```python
from build123d import *

# Parameters (mm, degrees)
BOSS_EXTRU_2_DEPTH      = 73
ESQUISSE6_W             = 6
ESQUISSE6_H             = 5
ENL_V_MAT_EXTRU_3_DEPTH = 83.675570757
ESQUISSE7_R             = 1.75
ENL_V_MAT_EXTRU_4_DEPTH = 12
ENL_V_START             = -12
ESQUISSE8_R             = 1.75
ENL_V_MAT_EXTRU_5_DEPTH = 12
CONG_1_R                = 3
ENL_V_START_2           = -3
ENL_V_MAT_EXTRU_6_DEPTH = 2.6
ENL_V_START_3           = -5.6
ENL_V_MAT_EXTRU_7_DEPTH = 2.6


with BuildPart() as part:
    # Esquisse3 → Boss.-Extru.2 (new body)
    with BuildSketch(Plane.XY):
        with BuildLine():
            ThreePointArc((-5, 37.165171868), (0, 37.5), (5, 37.165171868))
            Line((5, 37.165171868), (5, 29.580398915))
            Line((5, 29.580398915), (-5, 29.580398915))
            Line((-5, 29.580398915), (-5, 37.165171868))
        make_face()
    extrude(amount=BOSS_EXTRU_2_DEPTH)

    # Esquisse6 → Enlèv. mat.-Extru.3 (cut, through all)
    with BuildSketch(Plane.ZY.offset(5)):
        with Locations((18, 37.080398915)):
            Rectangle(ESQUISSE6_W, ESQUISSE6_H)
        with Locations((55, 37.080398915)):
            Rectangle(ESQUISSE6_W, ESQUISSE6_H)
    extrude(amount=-ENL_V_MAT_EXTRU_3_DEPTH, mode=Mode.SUBTRACT)

    # Esquisse7 → Enlèv. mat.-Extru.4 (cut)
    with BuildSketch(Plane.XY.offset(73)):
        with Locations((0, 33.75)):
            Circle(ESQUISSE7_R)
    extrude(amount=-ENL_V_MAT_EXTRU_4_DEPTH, mode=Mode.SUBTRACT)

    # Esquisse8 → Enlèv. mat.-Extru.5 (cut)
    with BuildSketch(Plane(origin=(0, 0, 0), x_dir=(-1, 0, 0), z_dir=(0, 0, -1)).offset(ENL_V_START)):
        with Locations(Location((0, 33.75, 0), (0, 0, 180))):
            Circle(ESQUISSE8_R)
    extrude(amount=ENL_V_MAT_EXTRU_5_DEPTH, mode=Mode.SUBTRACT)

    # Congé1
    cong_1_edges = [part.edges().sort_by_distance(p)[0] for p in [
        (5, 34.580398915, 18),
        (-5, 34.580398915, 18),
        (5, 34.580398915, 55),
        (-5, 34.580398915, 55),
    ]]
    fillet(cong_1_edges, radius=CONG_1_R)

    # Esquisse9 → Enlèv. mat.-Extru.6 (cut)
    with BuildSketch(Plane(origin=(0, 0, 0), x_dir=(-1, 0, 0), z_dir=(0, 0, -1)).offset(ENL_V_START_2)):
        with BuildLine():
            Line((-2.85, 37.391543162), (-2.85, 31.995448267))
            Line((-2.85, 31.995448267), (0, 30.35))
            Line((0, 30.35), (2.85, 31.995448267))
            Line((2.85, 31.995448267), (2.85, 37.391543162))
            ThreePointArc((2.85, 37.391543162), (0, 37.5), (-2.85, 37.391543162))
        make_face()
    extrude(amount=-ENL_V_MAT_EXTRU_6_DEPTH, mode=Mode.SUBTRACT)

    # Esquisse10 → Enlèv. mat.-Extru.7 (cut)
    with BuildSketch(Plane.XY.offset(73).offset(ENL_V_START_3)):
        with BuildLine():
            Line((-2.85, 37.391543162), (-2.85, 31.995448267))
            Line((-2.85, 31.995448267), (0, 30.35))
            Line((0, 30.35), (2.85, 31.995448267))
            Line((2.85, 31.995448267), (2.85, 37.391543162))
            ThreePointArc((2.85, 37.391543162), (0, 37.5), (-2.85, 37.391543162))
        make_face()
    extrude(amount=ENL_V_MAT_EXTRU_7_DEPTH, mode=Mode.SUBTRACT)


solid = part.part
```
Geometry: final body of the model. Coordinates: model frame, mm. A direction names the side the tool comes from. Round coordinates to 2 decimals unless told otherwise and drop trailing zeros. Loops run counter-clockwise (first coordinate to the right, second up) from the corner with the lowest first, then second, coordinate; pieces in that order, holes last.
Item 1: Mould query, pull axis X, two halves, no side actions, for faces 1 (the cylindrical face through (4.145, 33.678, 17.958)), 2 (the flat face through (0, 36, 52)), 3 (the flat face through (1.44, 31.18, 4.28)). Classes: released by +X, released by -X, zero draft, split by the parting line, or undercut.
Checked values:
face 1: released by +X
face 2: zero draft
face 3: undercut
Item 2: Line query: L1, parallel to Z at x = 2, y = 36.25; L2, parallel to Z at x = 0, y = 31.75; L3, parallel to Z at x = 4.25, y = 35.25. Output: solid intervals per line, ascending.
Checked values:
L1: z = 0 to 3, 5.6 to 15, 21 to 52, 58 to 67.4, 70 to 73
L2: z = 0 to 3, 5.6 to 67.4, 70 to 73
L3: z = 0 to 15, 21 to 52, 58 to 73
Item 3: Section A-A, the plane z = 68. Output: boundary loops of the cut face in (x, y).
Checked values:
outline: (-5, 29.58) - (5, 29.58) - (5, 37.17) arc R37.5 ccw to (2.85, 37.39) - (2.85, 32) - (0, 30.35) - (-2.85, 32) - (-2.85, 37.39) arc R37.5 ccw to (-5, 37.17) - close
Item 4: Contact query for flat-ended pins moving along their axis: P1, Ø1.2, axis at x = 0, z = 54.5, coming from the +Y side; P2, Ø2, axis at x = 2, z = 65, coming from the +Y side; P3, Ø1, axis at x = -2.5, y = 34, coming from the -Z side; P4, Ø2, axis at x = 0, y = 33.75, coming from the -Z side. Output: stop coordinate, or through.
Checked values:
P1: stops at y = 34.58
P2: stops at y = 37.49
P3: stops at z = 0
P4: stops at z = 12
Item 5: Reachability of faces 4 (the cylindrical face through (1.669, 33.224, 8.845)), 5 (the cylindrical face through (-4.145, 33.678, 18.042)), 6 (the flat face through (0, 36, 5.6)), 7 (the cylindrical face through (1.669, 34.276, 71.521)) from +Z, -Z, +X, -X, +Y, -Y: full face, straight path, thin tool, end or side. Return the list, or none.
Checked values:
face 4: -Z
face 5: -X, +Y
face 6: +Y
face 7: +Z
Item 6: Section B-B, the plane x = 1. State how many separate pieces and enclosed holes the cut face has, plus the area to 3 significant figures.
Checked values:
separate pieces: 3
enclosed holes: 0
area: 454 mm2
